Geometry check sheet. Reference: the model listing, model coordinates, mm. Coordinates: 2 decimals unless noted, no trailing zeros. Loops run counter-clockwise (first coordinate to the right, second up) from the corner with the lowest first, then second, coordinate; pieces in that order, holes last.
from build123d import *

# Parameters (mm, degrees)
SKETCH1_R           = 37.5
BOSS_EXTRUDE1_DEPTH = 5
SKETCH9_R           = 1.25
SKETCH9_R_2         = 1.5
SKETCH9_W           = 16
SKETCH9_H           = 20
SKETCH9_W_2         = 5
SKETCH9_H_2         = 5
CUT_EXTRUDE5_DEPTH  = 54.268189382


with BuildPart() as part:
    # Sketch1 → Boss-Extrude1 (new body)
    with BuildSketch(Plane.XY):
        Circle(SKETCH1_R)
    extrude(amount=BOSS_EXTRUDE1_DEPTH)

    # Sketch9 → Cut-Extrude5 (cut, through all)
    with BuildSketch(Plane.XY.offset(5)):
        with Locations((0, 30)):
            Circle(SKETCH9_R)
        with Locations((12.990381057, -7.5)):
            Circle(SKETCH9_R)
        with Locations((-12.990381057, -7.5)):
            Circle(SKETCH9_R)
        with Locations((20, 17.5)):
            Circle(SKETCH9_R_2)
        with Locations((-20, 17.5)):
            Circle(SKETCH9_R_2)
        with Locations(Location((20, -17.5, 0), (0, 0, 90))):
            Circle(SKETCH9_R_2)
        with Locations(Location((-20, -17.5, 0), (0, 0, 90))):
            Circle(SKETCH9_R_2)
        with Locations((0, 18)):
            Rectangle(SKETCH9_W, SKETCH9_H)
        with Locations((12.5, 17.5)):
            Rectangle(SKETCH9_W_2, SKETCH9_H_2)
        with Locations((27.5, 17.5)):
            Rectangle(SKETCH9_W_2, SKETCH9_H_2)
        with Locations((-27.5, 17.5)):
            Rectangle(SKETCH9_W_2, SKETCH9_H_2)
        with Locations((-12.5, 17.5)):
            Rectangle(SKETCH9_W_2, SKETCH9_H_2)
        with Locations((12.5, -17.5)):
            Rectangle(SKETCH9_W_2, SKETCH9_H_2)
        with Locations((27.5, -17.5)):
            Rectangle(SKETCH9_W_2, SKETCH9_H_2)
        with Locations((-27.5, -17.5)):
            Rectangle(SKETCH9_W_2, SKETCH9_H_2)
        with Locations((-12.5, -17.5)):
            Rectangle(SKETCH9_W_2, SKETCH9_H_2)
    extrude(amount=-CUT_EXTRUDE5_DEPTH, mode=Mode.SUBTRACT)


solid = part.part
(1) Sectioned sample at D-D on y = 17.5. State how many separate pieces and enclosed holes the cut face has, and give its area (3 significant figures).
Findings:
separate pieces: 8
enclosed holes: 0
area: 122 mm2
(2) Draft check along X on faces 1 (the flat face through (-8, 18, 3)), 2 (the cylindrical face through (-4.88, 37.18, 2.46)). Enter one of: +X half, -X half, draft (parallel to the pull), parting line (faces both ways), or undercut.
Findings:
face 1: undercut
face 2: parting line
(3) Sectioned sample at C-C on x = -20. Record the cut outline in (y, z), and give its area (3 significant figures).
Findings:
outline: (-31.72, 0) - (-19, 0) - (-19, 5) - (-31.72, 5) - close; (-16, 0) - (16, 0) - (16, 5) - (-16, 5) - close; (19, 0) - (31.72, 0) - (31.72, 5) - (19, 5) - close
area: 287 mm2
(4) Gauge pin test, flat ends, axial feed: pin 1 Ø2 at (y, z) = (-18, 3.5) entering from +X; pin 2 Ø3 at (y, z) = (-10.5, 1.5) entering from +X; pin 3 Ø2.5 at (x, z) = (13, 1.5) entering from -Y. Record the tip position at first contact, or that the pin passes through.
Findings:
pin 1: stops at x = 33.43
pin 2: stops at x = 36.4
pin 3: stops at y = -35.61
(5) Sectioned sample at A-A on y = 30. Record the cut outline in (x, z).
Findings:
outline: (-22.5, 0) - (-1.25, 0) - (-1.25, 5) - (-22.5, 5) - close; (1.25, 0) - (22.5, 0) - (22.5, 5) - (1.25, 5) - close
(6) Sectioned sample at B-B on y = -17.5. Record the cut outline in (x, z).
Findings:
outline: (-33.17, 0) - (-30, 0) - (-30, 5) - (-33.17, 5) - close; (-25, 0) - (-21.5, 0) - (-21.5, 5) - (-25, 5) - close; (-18.5, 0) - (-15, 0) - (-15, 5) - (-18.5, 5) - close; (-10, 0) - (10, 0) - (10, 5) - (-10, 5) - close; (15, 0) - (18.5, 0) - (18.5, 5) - (15, 5) - close; (21.5, 0) - (25, 0) - (25, 5) - (21.5, 5) - close; (30, 0) - (33.17, 0) - (33.17, 5) - (30, 5) - close
(7) Scan lines: L1, parallel to Y at x = 0, z = 1.9; L2, parallel to Y at x = 13.5, z = 0.35; L3, parallel to Y at x = -1, z = 3.25. Record each from-to range of solid material in increasing order.
Findings:
L1: y = -37.5 to 8, 28 to 28.75, 31.25 to 37.5
L2: y = -34.99 to -20, -15 to -8.64, -6.36 to 15, 20 to 34.99
L3: y = -37.49 to 8, 28 to 29.25, 30.75 to 37.49
